Work out the finished part from the listing and answer in its coordinate system (mm). Face numbers are marked on the shaded views. A direction names the side the tool comes from. Give positions to 0.01 mm unless a question says otherwise; leave off trailing zeros. Order: outer loops, then holes, each group sorted by start corner. A loop starts at its lowest first (then second) coordinate and runs counter-clockwise, first axis right, second up. Notation, with made-up numbers: (28, 52) -> (67, 52) arc R36 ccw to (67, 87) -> close; hole circle Ø7 at (14.25, 61). An arc over 180 degrees is marked (long way). Answer as CSV lines item,"result". Start each with the question number.
1. A cutting plane is placed at C-C (z = -17). Give the vertices of the cut face in (x, y).
2. Find the intervals of material crossed by L1, parallel to X at y = 9.5, z = -11.5; L2, parallel to Z at x = 10.5, y = 8, in increasing order.
3. For a pull along X with two mould halves and no side action, classify the marked faces 3, 4 and 5 as released by +X, released by -X, zero draft, split by the parting line, or undercut.
4. For the marked faces 1 and 2, determine the directions among +Z, -Z, +X, -X, +Y, -Y from which every point of the face is accessible in a straight line to the end or side of a thin tool.
5. A cutting plane is placed at B-B (z = -44). Give the vertices of the cut face in (x, y), then the cut area to 3 significant figures.
6. Flat-ended cylindrical pins translate along their axes: pin 1 (6 mm diameter, centred on y = 0, z = -44, fed in from -X); pin 2 (5 mm diameter, centred on x = 9.5, y = -15, fed in from -Z); pin 3 (8.5 mm diameter, centred on y = 0, z = -44, fed in from +X). Find the tip coordinate at first contact, or state that the pin passes through.
7. A cutting plane is placed at D-D (x = 21.5). Give the vertices of the cut face in (y, z), then the cut area to 3 significant figures.
8. A cutting plane is placed at A-A (y = 0). Give the vertices of the cut face in (x, z).
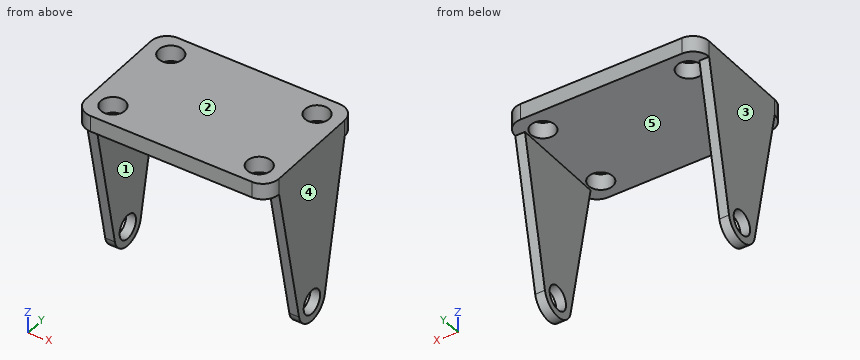
from build123d import *

# Parameters (mm, degrees)
F0_W     = 60
F0_H     = 40
F0_R     = 3.75
F1_DEPTH = 5
F2_R     = 5
F3_R     = 3.75
F4_DEPTH = 3


with BuildPart() as f1:
    # F0 (on Top) → F1 (new body)
    with BuildSketch(Plane.XY):
        Rectangle(F0_W, F0_H)
        with Locations((-22.647429, -13.222116)):
            Circle(F0_R, mode=Mode.SUBTRACT)
        with Locations((22.647429, -13.222116)):
            Circle(F0_R, mode=Mode.SUBTRACT)
        with Locations((-22.647429, 13.222116)):
            Circle(F0_R, mode=Mode.SUBTRACT)
        with Locations((22.647429, 13.222116)):
            Circle(F0_R, mode=Mode.SUBTRACT)
    extrude(amount=F1_DEPTH)

    # F2
    f2_edges = [f1.edges().sort_by_distance(p)[0] for p in [
        (-30, -20, 2.5),
        (30, -20, 2.5),
        (30, 20, 2.5),
        (-30, 20, 2.5),
    ]]
    fillet(f2_edges, radius=F2_R)

    # F3 (on face) → F4 (join)
    with BuildSketch(Plane.YZ.offset(30)):
        with BuildLine():
            Line((15, 0), (-15, 0))
            Line((-15, 0), (-5.881443, -45.186856))
            ThreePointArc((-5.881443, -45.186856), (0, -50), (5.881443, -45.186856))
            Line((5.881443, -45.186856), (15, 0))
        make_face()
        with Locations((0, -44)):
            Circle(F3_R, mode=Mode.SUBTRACT)
    extrude(amount=-F4_DEPTH)

    # F5: F1 across plane


with BuildPart() as f1_1:
    add(f1.part)
    add(f1.part.mirror(Plane.YZ))


solid = f1_1.part
Answer sheet:
1,outline,"(-30, -11.57) -> (-27, -11.57) -> (-27, 11.57) -> (-30, 11.57) -> close; (27, -11.57) -> (30, -11.57) -> (30, 11.57) -> (27, 11.57) -> close"
2,L1,"x = -30 to -27, 27 to 30"
2,L2,"z = 0 to 5"
3,face 3,"released by -X"
3,face 4,"released by +X"
3,face 5,"undercut"
4,face 1,"-Z, +Y, -Y"
4,face 2,"+Z, +X, -X, +Y, -Y"
5,outline,"(-30, -6.12) -> (-27, -6.12) -> (-27, -3.75) -> (-30, -3.75) -> close; (-30, 3.75) -> (-27, 3.75) -> (-27, 6.12) -> (-30, 6.12) -> close; (27, -6.12) -> (30, -6.12) -> (30, -3.75) -> (27, -3.75) -> close; (27, 3.75) -> (30, 3.75) -> (30, 6.12) -> (27, 6.12) -> close"
5,area,"28.5 mm^2"
6,pin 1,"passes through"
6,pin 2,"stops at z = 0"
6,pin 3,"stops at x = 30"
7,outline,"(-20, 0) -> (-16.79, 0) -> (-16.79, 5) -> (-20, 5) -> close; (-9.65, 0) -> (9.65, 0) -> (9.65, 5) -> (-9.65, 5) -> close; (16.79, 0) -> (20, 0) -> (20, 5) -> (16.79, 5) -> close"
7,area,"129 mm^2"
8,outline,"(-30, -50) -> (-27, -50) -> (-27, -47.75) -> (-30, -47.75) -> close; (-30, -40.25) -> (-27, -40.25) -> (-27, 0) -> (27, 0) -> (27, -40.25) -> (30, -40.25) -> (30, 5) -> (-30, 5) -> close; (27, -50) -> (30, -50) -> (30, -47.75) -> (27, -47.75) -> close"
